Part model, mm, in its own coordinate system. A direction names the side the tool comes from. Coordinates: 2 decimals unless noted, no trailing zeros. Write each loop counter-clockwise with the first axis right and the second up, starting at its lowest first coordinate (ties: lowest second). Pieces come first, ordered by that corner, then holes. Notation, with made-up numbers: (46.5, 59) - (56.5, 59) arc R20 ccw to (56.5, 91) - close; hole circle Ø2 at (-28.5, -36). An arc over 180 degrees is marked (long way). Use a Markdown table: item, result.
```python
from build123d import *

# Parameters (mm, degrees)
F0_R     = 4.474653
F0_R_2   = 8.455693
F0_R_3   = 6.210572
F1_DEPTH = 12.7
F2_DEPTH = 12.7


with BuildPart() as f1:
    # F0 (on Front) → F1 (new body)
    with BuildSketch(Plane.XZ):
        Polygon((41.521776, 47.588885), (-9.669455, 47.588885), (-9.669455, 21.803673), (-14.030189, 21.803673), (-14.030189, 10.048649), (-31.093935, -28.818769), (3.223152, -28.818769), (3.223152, -16.115759), (50.243247, -16.115759), (67.117393, 0), (67.117393, 30.904336), (41.521776, 30.904336), align=None)
        with Locations((-12.693984, -15.35737)):
            Circle(F0_R, mode=Mode.SUBTRACT)
        with Locations((33.378128, -3.412749)):
            Circle(F0_R_2, mode=Mode.SUBTRACT)
        with Locations((18.390924, 28.060379)):
            Circle(F0_R_3, mode=Mode.SUBTRACT)
    extrude(amount=F1_DEPTH)

    # F0 (on Front) → F2 (join)
    with BuildSketch(Plane.XZ):
        Polygon((41.521776, 47.588885), (-9.669455, 47.588885), (-9.669455, 21.803673), (-14.030189, 21.803673), (-14.030189, 10.048649), (-31.093935, -28.818769), (3.223152, -28.818769), (3.223152, -16.115759), (50.243247, -16.115759), (67.117393, 0), (67.117393, 30.904336), (41.521776, 30.904336), align=None)
        with Locations((-12.693984, -15.35737)):
            Circle(F0_R, mode=Mode.SUBTRACT)
        with Locations((33.378128, -3.412749)):
            Circle(F0_R_2, mode=Mode.SUBTRACT)
        with Locations((18.390924, 28.060379)):
            Circle(F0_R_3, mode=Mode.SUBTRACT)
    extrude(amount=F2_DEPTH)


solid = f1.part
```
Item 1: Two-plate mould, pull along X, no slides. Class faces 1 (the face through (17, -12.7, 10)), 2 (the face through (-13.664, -6.261, -19.726)), 3 (the face through (-14.03, -6, 16)): pulls with the +X half, pulls with the -X half, needs draft (parallel to the pull), parting line crosses it, or undercut.
From the geometry:
| item | result |
|---|---|
| face 1 | needs draft |
| face 2 | undercut |
| face 3 | pulls with the -X half |
Item 2: Band-saw the part on C-C, the plane y = -11. Give the cut face in (x, z), then the cut area to 3 significant figures.
From the geometry:
| item | result |
|---|---|
| outline | (-31.09, -28.82) - (3.22, -28.82) - (3.22, -16.12) - (50.24, -16.12) - (67.12, 0) - (67.12, 30.9) - (41.52, 30.9) - (41.52, 47.59) - (-9.67, 47.59) - (-9.67, 21.8) - (-14.03, 21.8) - (-14.03, 10.05) - close; hole circle Ø8.95 at (-12.69, -15.36); hole circle Ø12.42 at (18.39, 28.06); hole circle Ø16.91 at (33.38, -3.41) |
| area | 4,640 mm^2 |
Item 3: Drill centre lines: probe 1 along Z at (x, y) = (38.5, -10); probe 2 along X at (y, z) = (-1.75, 10); probe 3 along X at (y, z) = (-2, -15.5). Where is each one in solid material? Low to high.
From the geometry:
| item | result |
|---|---|
| probe 1 | -16.12 to -10.14, 3.32 to 47.59 |
| probe 2 | -14.05 to 67.12 |
| probe 3 | -25.25 to -17.17, -8.22 to 50.89 |
Item 4: Which spindle directions (+Z, -Z, +X, -X, +Y, -Y) get a long thin tool onto all of the face, cutting with end or side? Do faces 4 (the face through (-14, -6, -28.819)), 5 (the face through (-9.669, -6, 35)), 6 (the face through (3.223, -6, -23)), 7 (the face through (17, 0, 10)), 8 (the face through (41.522, -6, 39)). Say none if no direction does.
From the geometry:
| item | result |
|---|---|
| face 4 | -Z, +X, -X, +Y, -Y |
| face 5 | +Z, -X, +Y, -Y |
| face 6 | -Z, +X, +Y, -Y |
| face 7 | +Z, -Z, +X, -X, +Y |
| face 8 | +Z, +X, +Y, -Y |
Item 5: Band-saw the part on A-A, the plane x = 35. Give the cut face in (y, z).
From the geometry:
| item | result |
|---|---|
| outline | (-12.7, -16.12) - (0, -16.12) - (0, -11.71) - (-12.7, -11.71) - close; (-12.7, 4.89) - (0, 4.89) - (0, 47.59) - (-12.7, 47.59) - close |
Item 6: Drop flat-ended pins along their axis: P1, Ø4, axis at y = -7.5, z = 36.5, coming from the +X side; P2, Ø6.5, axis at x = 50.5, y = -9, coming from the +Z side; P3, Ø5, axis at y = -9.5, z = 37.5, coming from the -X side. Give the stop position or say it passes through.
From the geometry:
| item | result |
|---|---|
| P1 | x = 41.52 |
| P2 | z = 30.9 |
| P3 | x = -9.67 |
Item 7: Band-saw the part on D-D, the plane x = 8. Give the cut face in (y, z), then the cut area to 3 significant figures.
From the geometry:
| item | result |
|---|---|
| outline | (-12.7, -16.12) - (0, -16.12) - (0, 47.59) - (-12.7, 47.59) - close |
| area | 809 mm^2 |
Item 8: Band-saw the part on B-B, the plane z = 27. Give the cut face in (x, y), then the cut area to 3 significant figures.
From the geometry:
| item | result |
|---|---|
| outline | (-9.67, -12.7) - (12.27, -12.7) - (12.27, 0) - (-9.67, 0) - close; (24.51, -12.7) - (67.12, -12.7) - (67.12, 0) - (24.51, 0) - close |
| area | 820 mm^2 |
